```python
from build123d import *

# Parameters (mm, degrees)
F0_R     = 1.6
F0_W     = 2.7
F0_H     = 4
F0_H_2   = 4.2
F1_DEPTH = 2.5


with BuildPart() as f1:
    # F0 (on Front) → F1 (new body)
    with BuildSketch(Plane.XZ):
        with BuildLine():
            Line((-72.446153, 21), (-100, 0))
            Line((-100, 0), (-95.938877, 0))
            ThreePointArc((-95.938877, 0), (-95.657736, 0.024894), (-95.376595, 0))
            Line((-95.376595, 0), (0, 0))
            Line((0, 0), (0, 21))
            Line((0, 21), (-15.5, 21))
            Line((-15.5, 21), (-72.446153, 21))
        make_face()
        with Locations((-56.57779, 10)):
            Circle(F0_R, mode=Mode.SUBTRACT)
        with Locations((-23, 10)):
            Circle(F0_R, mode=Mode.SUBTRACT)
        with BuildLine():
            Line((-95.938877, 0), (-100, 0))
            Line((-100, 0), (-100, -13.5))
            ThreePointArc((-100, -13.5), (-97.803301, -18.803301), (-92.5, -21))
            Line((-92.5, -21), (0, -21))
            Line((0, -21), (0, -19))
            Line((0, -19), (-1.515, -19))
            Line((-1.515, -19), (-1.515, -15))
            Line((-1.515, -15), (0, -15))
            Line((0, -15), (0, 0))
            Line((0, 0), (-95.376595, 0))
            ThreePointArc((-95.376595, 0), (-94.430987, -0.547932), (-94.057736, -1.575106))
            ThreePointArc((-94.057736, -1.575106), (-96.68491, -2.801855), (-95.938877, 0))
        make_face()
        Polygon((-92.175341, -14.942273), (-89.638171, -14.018818), (-88.201686, -17.965527), (-90.738856, -18.888982), align=None, mode=Mode.SUBTRACT)
        with Locations((-72.47779, -17.245993)):
            Circle(F0_R, mode=Mode.SUBTRACT)
        with Locations((-15.465, -17)):
            Rectangle(F0_W, F0_H, mode=Mode.SUBTRACT)
        with Locations((-10.365, -17)):
            Rectangle(F0_W, F0_H, mode=Mode.SUBTRACT)
        with Locations((-5.265, -17)):
            Rectangle(F0_W, F0_H, mode=Mode.SUBTRACT)
        with Locations((-91.32779, -10)):
            Rectangle(F0_W, F0_H_2, mode=Mode.SUBTRACT)
        Polygon((-87.47779, -12.1), (-87.47779, -7.9), (-72.534475, -7.9), (-59.065768, -2.997792), (-57.697688, -6.756562), (-60.839257, -7.9), (-57.47779, -7.9), (-57.47779, -12.1), (-72.378662, -12.1), (-85.888466, -17.017167), (-87.256547, -13.258396), (-84.07388, -12.1), align=None, mode=Mode.SUBTRACT)
        with Locations((-53.62779, -10)):
            Rectangle(F0_W, F0_H_2, mode=Mode.SUBTRACT)
        Polygon((-56.748929, -2.048113), (-54.211759, -1.124659), (-52.775274, -5.071368), (-55.312444, -5.994822), align=None, mode=Mode.SUBTRACT)
        with Locations((-23, -8.5)):
            Circle(F0_R, mode=Mode.SUBTRACT)
        with BuildLine():
            Line((62.46032, 0), (0, 0))
            Line((0, 0), (0, -15))
            Line((0, -15), (1.185, -15))
            Line((1.185, -15), (1.185, -19))
            Line((1.185, -19), (0, -19))
            Line((0, -19), (0, -21))
            Line((0, -21), (15.5, -21))
            Line((15.5, -21), (40.587112, -2.866724))
            Line((40.587112, -2.866724), (85, -2.866724))
            ThreePointArc((85, -2.866724), (89.636856, -2.132052), (93.819502, 0))
            Line((93.819502, 0), (85.53968, 0))
            ThreePointArc((85.53968, 0), (84, -1.164814), (82.46032, 0))
            Line((82.46032, 0), (65.53968, 0))
            ThreePointArc((65.53968, 0), (64, -1.164814), (62.46032, 0))
        make_face()
        with Locations((4.935, -17)):
            Rectangle(F0_W, F0_H, mode=Mode.SUBTRACT)
        with Locations((10.035, -17)):
            Rectangle(F0_W, F0_H, mode=Mode.SUBTRACT)
        with Locations((19, -8.5)):
            Circle(F0_R, mode=Mode.SUBTRACT)
        with BuildLine():
            Line((0, 21), (0, 0))
            Line((0, 0), (62.46032, 0))
            ThreePointArc((62.46032, 0), (63.780327, 2.020034), (65.6, 0.435186))
            ThreePointArc((65.6, 0.435186), (65.584848, 0.215513), (65.53968, 0))
            Line((65.53968, 0), (82.46032, 0))
            ThreePointArc((82.46032, 0), (83.780327, 2.020034), (85.6, 0.435186))
            ThreePointArc((85.6, 0.435186), (85.584848, 0.215513), (85.53968, 0))
            Line((85.53968, 0), (93.819502, 0))
            ThreePointArc((93.819502, 0), (98.365862, 5.324918), (100, 12.133276))
            Line((100, 12.133276), (100, 21))
            Line((100, 21), (0, 21))
        make_face()
        with BuildLine():
            Line((18, 7.460512), (42, 7.460512))
            ThreePointArc((42, 7.460512), (42.353553, 7.314066), (42.5, 6.960512))
            Line((42.5, 6.960512), (42.5, 5.460512))
            ThreePointArc((42.5, 5.460512), (42.353553, 5.106959), (42, 4.960512))
            Line((42, 4.960512), (18, 4.960512))
            ThreePointArc((18, 4.960512), (17.646447, 5.106959), (17.5, 5.460512))
            Line((17.5, 5.460512), (17.5, 6.960512))
            ThreePointArc((17.5, 6.960512), (17.646447, 7.314066), (18, 7.460512))
        make_face(mode=Mode.SUBTRACT)
        Polygon((56.752226, 2.039054), (54.215056, 1.115599), (52.778572, 5.062308), (55.315742, 5.985763), align=None, mode=Mode.SUBTRACT)
        with Locations((53.62779, 10)):
            Rectangle(F0_W, F0_H_2, mode=Mode.SUBTRACT)
        Polygon((57.47779, 8), (57.47779, 12.2), (72.389218, 12.2), (85.855752, 17.101418), (87.292237, 13.154709), (84.669196, 12.2), (87.47779, 12.2), (87.47779, 8), (73.129791, 8), (59.101458, 2.894104), (57.664973, 6.840813), (60.849813, 8), align=None, mode=Mode.SUBTRACT)
        with Locations((91.32779, 10)):
            Rectangle(F0_W, F0_H_2, mode=Mode.SUBTRACT)
        with Locations((64, 16.5)):
            Circle(F0_R, mode=Mode.SUBTRACT)
        Polygon((88.204984, 17.956468), (90.742154, 18.879922), (92.178638, 14.933213), (89.641468, 14.009759), align=None, mode=Mode.SUBTRACT)
    extrude(amount=F1_DEPTH)


solid = f1.part
```
Here's how the part is built. I have some questions about the finished solid (model axes, mm). A direction names the side the tool comes from. Coordinates: 2 decimals unless noted, no trailing zeros. Loops run counter-clockwise (first coordinate to the right, second up) from the corner with the lowest first, then second, coordinate; pieces in that order, holes last. Notation, with made-up numbers: (86, 20) - (123, 20) arc R33 ccw to (123, 56) - close; hole circle Ø7 at (82.5, 31). An arc over 180 degrees is marked (long way). Return JSON: item names as keys, results as strings. Group by question number.
Item 1: If we section it at A-A on x = 70: Write out the boundary of the cut face in (y, z).
Item 2: If we section it at C-C on x = 45.5: Write out the boundary of the cut face in (y, z).
Item 3: I need wall thicknesses on line 1 (Z direction, x = -23, y = -1.7); line 2 (Z direction, x = 64, y = -0.6); line 3 (X direction, y = -2.1, z = 9). Which ranges of each line are inside material? Lowest first, please. Write a range as from..to.
Item 4: Will these pins go through, and if not, where does the flat tip stop? P1, Ø1.2, axis at y = -1, z = 6, coming from the -X side; P2, Ø1.2, axis at y = -1, z = 10.5, coming from the -X side; P3, Ø0.8, axis at y = -1, z = 10.5, coming from the -X side.
Item 5: If we section it at B-B on y = -1.85: State how many separate pieces and enclosed holes the cut face has, and give its area (3 significant figures).
Item 6: On a 3-axis mill with a long thin cutter (end or side, diameter ignored), from which of +Z, -Z, +X, -X, +Y, -Y can I reach the whole of each face in a straight line? I mean faces 4 (the face through (66.21, -1.23, 5.48)), 5 (the face through (-1, 0, 5)). Say none if no direction works.
Item 7: We'd pull the mould along X, two halves only. Please class faces 1 (the face through (27.87, -1.23, -12.06)), 2 (the face through (-65.89, -1.23, -5.48)), 3 (the face through (-1, -2.5, 5)): +X half, -X half, draft (parallel to the pull), parting line (faces both ways), or undercut.
Calculated:
{
 "1": {"outline": "(-2.5, -2.87) - (0, -2.87) - (0, 6.86) - (-2.5, 6.86) - close; (-2.5, 12.2) - (0, 12.2) - (0, 21) - (-2.5, 21) - close"},
 "2": {"outline": "(-2.5, -2.87) - (0, -2.87) - (0, 21) - (-2.5, 21) - close"},
 "3": {"line 1": "z = -21..-10.1, -6.9..8.4, 11.6..21", "line 2": "z = -2.87..-1.16, 2.04..4.68, 12.2..14.9, 18.1..21", "line 3": "x = -88.19..-57.83, -55.33..-24.25, -21.75..52.28, 54.98..57.48, 87.48..89.98, 92.68..99.67"},
 "4": {"P1": "stops at x = -92.91", "P2": "stops at x = -87.01", "P3": "stops at x = -86.75"},
 "5": {"separate pieces": "1", "enclosed holes": "26", "area": "6,060 mm^2"},
 "6": {"face 4": "+Y, -Y", "face 5": "+Z, -Z, +X, -X, +Y"},
 "7": {"face 1": "+X half", "face 2": "undercut", "face 3": "draft"}
}
